```python
from build123d import *

# Parameters (mm, degrees)
SKETCH_1_W          = 32
SKETCH_1_H          = 321
EXTRUDE_1_DEPTH     = 5.5
SKETCH_2_R          = 1.05
SKETCH_2_W          = 25
SKETCH_2_H          = 18
CUT_EXTRUDE_1_DEPTH = 162.389280933
SKETCH_3_W          = 11
SKETCH_3_H          = 5.5
CUT_EXTRUDE_2_DEPTH = 162.389280933


with BuildPart() as part:
    # ｽｹｯﾁ1 → ﾎﾞｽ - 押し出し1 (new body)
    with BuildSketch(Plane.XY):
        Rectangle(SKETCH_1_W, SKETCH_1_H)
    extrude(amount=EXTRUDE_1_DEPTH)

    # ｽｹｯﾁ2 → ｶｯﾄ - 押し出し1 (cut, through all)
    with BuildSketch(Plane.XY.offset(5.5)):
        with Locations((12, 12)):
            Circle(SKETCH_2_R)
        with Locations((12, -12)):
            Circle(SKETCH_2_R)
        with Locations((-12, 12)):
            Circle(SKETCH_2_R)
        with Locations((-12, -12)):
            Circle(SKETCH_2_R)
        Rectangle(SKETCH_2_W, SKETCH_2_H)
    extrude(amount=-CUT_EXTRUDE_1_DEPTH, mode=Mode.SUBTRACT)

    # ｽｹｯﾁ3 → ｶｯﾄ - 押し出し2 (cut, through all)
    with BuildSketch(Plane.XY.offset(5.5)):
        with Locations((-10.5, 157.75)):
            Rectangle(SKETCH_3_W, SKETCH_3_H)
        with Locations((10.5, 157.75)):
            Rectangle(SKETCH_3_W, SKETCH_3_H)
        with Locations((10.5, -157.75)):
            Rectangle(SKETCH_3_W, SKETCH_3_H)
        with Locations((-10.5, -157.75)):
            Rectangle(SKETCH_3_W, SKETCH_3_H)
    extrude(amount=-CUT_EXTRUDE_2_DEPTH, mode=Mode.SUBTRACT)


solid = part.part
```
Model file for the job. Use its own axes, mm. A direction names the side the tool comes from. Coordinates: 2 decimals unless noted, no trailing zeros. Write each loop counter-clockwise with the first axis right and the second up, starting at its lowest first coordinate (ties: lowest second). Pieces come first, ordered by that corner, then holes. Notation, with made-up numbers: (58, 64.25) - (116, 64.25) arc R19 cw to (116, 77.25) - close; hole circle Ø9 at (70.5, 73.5). An arc over 180 degrees is marked (long way). Use a Markdown table: item, result. Add a question column.
Item 1: 3-axis set-ups, long thin cutter, end or side, ignore diameter. For faces 4 (the face through (-12.5, 0, 3)), 5 (the face through (10, -155, 3)), 6 (the face through (10, 155, 3)), 7 (the face through (-5, 158, 3)), 8 (the face through (-11, -155, 3)): which of +Z, -Z, +X, -X, +Y, -Y reach the whole face in a straight line?
Item 2: Drop a flat-ended pin along its axis: pin 1 (3 mm diameter, centred on x = 12, z = 2.5, fed in from -Y). Give the stop position or say it passes through.
Item 3: Drill centre lines: line 1 along Y through (x, z) = (-12, 2.6); line 2 along Y through (x, z) = (0.5, 3.95); line 3 along Y through (x, z) = (14, 4.1). Where is each one in solid material? Low to high.
Item 4: Band-saw the part on A-A, the plane x = 0. Write the cut outline in (y, z), and give its area (3 significant figures).
Item 5: Two-plate mould, pull along Y, no slides. Class faces 1 (the face through (0, -9, 3)), 2 (the face through (-5, -158, 3)), 3 (the face through (0, 160.5, 3)): pulls with the +Y half, pulls with the -Y half, needs draft (parallel to the pull), parting line crosses it, or undercut.
Item 6: Band-saw the part on B-B, the plane z = 2.8. Write the cut outline in (x, y), and give its area (3 significant figures).
A:
| question | item | result |
|---|---|---|
| 1 | face 4 | +Z, -Z |
| 1 | face 5 | +Z, -Z, +X, -Y |
| 1 | face 6 | +Z, -Z, +X, +Y |
| 1 | face 7 | +Z, -Z, -X, +Y |
| 1 | face 8 | +Z, -Z, -X, -Y |
| 2 | pin 1 | stops at y = -155 |
| 3 | line 1 | y = -155 to -13.05, -10.95 to -9, 9 to 10.95, 13.05 to 155 |
| 3 | line 2 | y = -160.5 to -9, 9 to 160.5 |
| 3 | line 3 | y = -155 to 155 |
| 4 | outline | (-160.5, 0) - (-9, 0) - (-9, 5.5) - (-160.5, 5.5) - close; (9, 0) - (160.5, 0) - (160.5, 5.5) - (9, 5.5) - close |
| 4 | area | 1,670 mm² |
| 5 | face 1 | undercut |
| 5 | face 2 | needs draft |
| 5 | face 3 | pulls with the +Y half |
| 6 | outline | (-16, -155) - (-5, -155) - (-5, -160.5) - (5, -160.5) - (5, -155) - (16, -155) - (16, 155) - (5, 155) - (5, 160.5) - (-5, 160.5) - (-5, 155) - (-16, 155) - close; hole circle Ø2.1 at (-12, -12); hole circle Ø2.1 at (-12, 12); hole (-12.5, -9) - (12.5, -9) - (12.5, 9) - (-12.5, 9) - close; hole circle Ø2.1 at (12, -12); hole circle Ø2.1 at (12, 12) |
| 6 | area | 9,570 mm² |
